For this review, take the finished solid that the model builds, in its own axes (mm). Face numbers are marked on the shaded views. A direction names the side the tool comes from. Give positions to 0.01 mm unless a question says otherwise; leave off trailing zeros. Write each loop counter-clockwise with the first axis right and the second up, starting at its lowest first coordinate (ties: lowest second). Pieces come first, ordered by that corner, then holes.
1) Wall thickness on line 1 along Z through (x, y) = (-4.5, 2.25); line 2 along Y through (x, z) = (6.5, 1); line 3 along X through (y, z) = (1, 4): over which ranges is each line inside the solid? List them lowest first.
2) We need section B-B on y = 0. Give the boundary of the cut face in (x, z) (3 decimals), and give its area (3 significant figures).
3) We need section A-A on z = 6. Give the boundary of the cut face in (x, y) (3 decimals), and give its area (3 significant figures).
4) We need section D-D on z = 4.5. Give the boundary of the cut face in (x, y) (3 decimals).
5) Draft analysis for pull direction Y (two halves, no side actions). For the marked faces 1, 2 and 3, state which applies: pulls with the +Y half, pulls with the -Y half, needs draft (parallel to the pull), parting line crosses it, or undercut.
6) For P1, Ø0.9, axis at x = 0, y = 1, coming from the +Z side; P2, Ø1, axis at x = 2.5, z = 4, coming from the -Y side; P3, Ø3, axis at y = 1.5, z = 6.5, coming from the -X side (3 decimals), all flat-tipped, find the tip position at first contact; note any pin that passes through.
7) Machinability: for the marked faces 4 and 5, which of the approach directions +Z, -Z, +X, -X, +Y, -Y give a long, thin tool a straight path to every point of the face, cutting with its end or side? Answer none if there is none.
8) We need section C-C on x = 0. Give the boundary of the cut face in (y, z) (3 decimals), and give its area (3 significant figures).
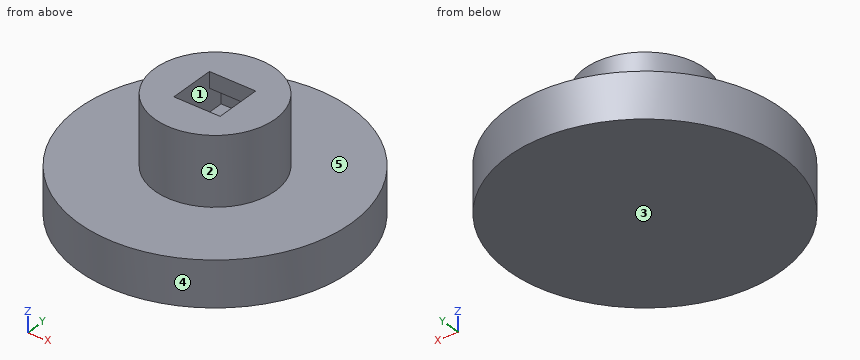
from build123d import *

# Parameters (mm, degrees)
F0_R     = 9
F1_DEPTH = 3
F2_R     = 3.975
F3_DEPTH = 4.5
F4_W     = 3.05
F4_H     = 3.05
F5_DEPTH = 2.55
F6_W     = 3.05
F6_H     = 1.5
F7_DEPTH = 1


with BuildPart() as f1:
    # F0 (on Top) → F1 (new body)
    with BuildSketch(Plane.XY):
        Circle(F0_R)
    extrude(amount=F1_DEPTH)

    # F2 (on face) → F3 (join)
    with BuildSketch(Plane.XY.offset(3)):
        Circle(F2_R)
    extrude(amount=F3_DEPTH)

    # F4 (on face) → F5 (cut)
    with BuildSketch(Plane.XY.offset(7.5)):
        with Locations((0, -0.025)):
            Rectangle(F4_W, F4_H)
    extrude(amount=-F5_DEPTH, mode=Mode.SUBTRACT)

    # F6 (on face) → F7 (cut)
    with BuildSketch(Plane.XZ.offset(-1.5)):
        with Locations((0, 5.7)):
            Rectangle(F6_W, F6_H)
    extrude(amount=-F7_DEPTH, mode=Mode.SUBTRACT)


solid = f1.part
Results list:
1. line 1: z = 0 to 3
1. line 2: y = -6.22 to 6.22
1. line 3: x = -3.85 to 3.85
2. outline: (-9, 0) - (9, 0) - (9, 3) - (3.975, 3) - (3.975, 7.5) - (1.525, 7.5) - (1.525, 4.95) - (-1.525, 4.95) - (-1.525, 7.5) - (-3.975, 7.5) - (-3.975, 3) - (-9, 3) - close
2. area: 82.0 mm2
3. outline: circle Ø7.95 at (0, 0); hole (-1.525, -1.55) - (1.525, -1.55) - (1.525, 2.5) - (-1.525, 2.5) - close
3. area: 37.3 mm2
4. outline: circle Ø7.95 at (0, 0)
5. face 1: undercut
5. face 2: parting line crosses it
5. face 3: needs draft
6. P1: stops at z = 4.95
6. P2: stops at y = -3.44
6. P3: stops at x = -3.975
7. face 4: +Z, -Z
7. face 5: +Z
8. outline: (-9, 0) - (9, 0) - (9, 3) - (3.975, 3) - (3.975, 7.5) - (1.5, 7.5) - (1.5, 6.45) - (2.5, 6.45) - (2.5, 4.95) - (-1.55, 4.95) - (-1.55, 7.5) - (-3.975, 7.5) - (-3.975, 3) - (-9, 3) - close
8. area: 80.5 mm2
